Geometry check sheet. Reference: the model listing, model coordinates, mm. Coordinates: 2 decimals unless noted, no trailing zeros. Loops run counter-clockwise (first coordinate to the right, second up) from the corner with the lowest first, then second, coordinate; pieces in that order, holes last. Notation, with made-up numbers: (35.25, -6.75) - (70.25, -6.75) arc R12 ccw to (70.25, 4.25) - close; hole circle Ø11 at (36, 29). An arc over 180 degrees is marked (long way). Write item = value, one per line. Start each with the question number.
from build123d import *

# Parameters (mm, degrees)
F0_R     = 1.6
F1_DEPTH = 3.175


# Not quite as in the source:
# - a length typed as a fraction of an inch, garbled in the dataset ("3 / 203.2 mm" for 3/8 in), is restored


with BuildPart() as f1:
    # F0 (on Front) → F1 (new body)
    with BuildSketch(Plane.XZ):
        with BuildLine():
            Line((27.46, 0), (2.54, 0))
            ThreePointArc((2.54, 0), (0.7439487758, -0.7439487758), (0, -2.54))
            Line((0, -2.54), (0, -77.46))
            ThreePointArc((0, -77.46), (0.7439487758, -79.2560512242), (2.54, -80))
            Line((2.54, -80), (27.46, -80))
            ThreePointArc((27.46, -80), (29.2560512242, -79.2560512242), (30, -77.46))
            Line((30, -77.46), (30, -2.54))
            ThreePointArc((30, -2.54), (29.2560512242, -0.7439487758), (27.46, 0))
        make_face()
        with Locations((5, -75)):
            Circle(F0_R, mode=Mode.SUBTRACT)
        with Locations((5, -65)):
            Circle(F0_R, mode=Mode.SUBTRACT)
        with Locations((15, -75)):
            Circle(F0_R, mode=Mode.SUBTRACT)
        with Locations((15, -65)):
            Circle(F0_R, mode=Mode.SUBTRACT)
        with Locations((5, -55)):
            Circle(F0_R, mode=Mode.SUBTRACT)
        with Locations((5, -45)):
            Circle(F0_R, mode=Mode.SUBTRACT)
        with Locations((15, -55)):
            Circle(F0_R, mode=Mode.SUBTRACT)
        with Locations((15, -45)):
            Circle(F0_R, mode=Mode.SUBTRACT)
        with Locations((25, -75)):
            Circle(F0_R, mode=Mode.SUBTRACT)
        with Locations((25, -65)):
            Circle(F0_R, mode=Mode.SUBTRACT)
        with Locations((25, -55)):
            Circle(F0_R, mode=Mode.SUBTRACT)
        with Locations((25, -45)):
            Circle(F0_R, mode=Mode.SUBTRACT)
        with Locations((5, -35)):
            Circle(F0_R, mode=Mode.SUBTRACT)
        with Locations((5, -25)):
            Circle(F0_R, mode=Mode.SUBTRACT)
        with Locations((15, -35)):
            Circle(F0_R, mode=Mode.SUBTRACT)
        with Locations((15, -25)):
            Circle(F0_R, mode=Mode.SUBTRACT)
        with Locations((5, -15)):
            Circle(F0_R, mode=Mode.SUBTRACT)
        with Locations((5, -5)):
            Circle(F0_R, mode=Mode.SUBTRACT)
        with Locations((15, -15)):
            Circle(F0_R, mode=Mode.SUBTRACT)
        with Locations((15, -5)):
            Circle(F0_R, mode=Mode.SUBTRACT)
        with Locations((25, -35)):
            Circle(F0_R, mode=Mode.SUBTRACT)
        with Locations((25, -25)):
            Circle(F0_R, mode=Mode.SUBTRACT)
        with Locations((25, -15)):
            Circle(F0_R, mode=Mode.SUBTRACT)
        with Locations((25, -5)):
            Circle(F0_R, mode=Mode.SUBTRACT)
    extrude(amount=F1_DEPTH)


solid = f1.part
(1) Draft check along X on faces 1 (the face through (30, -2, -41)), 2 (the face through (24.65, -1.57, -36.56)), 3 (the face through (15, -3.175, -39)). Enter one of: pulls with the +X half, pulls with the -X half, needs draft (parallel to the pull), parting line crosses it, or undercut.
(2) Scan lines: line 1 (X direction, y = -1.4, z = -75); line 2 (X direction, y = -0.4, z = -66); line 3 (Z direction, x = 28.75, y = -0.75). Record each from-to range of solid material in increasing order.
(3) Sectioned sample at A-A on z = -65. Enter the section's corners in (x, y) (3 decimals).
(4) Sectioned sample at B-B on x = 15. Count the separate pieces of the cut face and the enclosed holes in it, plus the area to 3 significant figures.
(5) Depth check by flat-ended pin: pin 1 (3 mm diameter, centred on x = 25, z = -25, fed in from -Y). Enter the tip coordinate at first touch or a pass-through.
Working result:
q1.face_1 = pulls with the +X half
q1.face_2 = undercut
q1.face_3 = needs draft
q2.line_1 = 0 to 3.4, 6.6 to 13.4, 16.6 to 23.4, 26.6 to 30
q2.line_2 = 0 to 3.75, 6.25 to 13.75, 16.25 to 23.75, 26.25 to 30
q2.line_3 = -79.65 to -0.35
q3.outline = (0, -3.175) - (3.4, -3.175) - (3.4, 0) - (0, 0) - close; (6.6, -3.175) - (13.4, -3.175) - (13.4, 0) - (6.6, 0) - close; (16.6, -3.175) - (23.4, -3.175) - (23.4, 0) - (16.6, 0) - close; (26.6, -3.175) - (30, -3.175) - (30, 0) - (26.6, 0) - close
q4.separate_pieces = 9
q4.enclosed_holes = 0
q4.area = 173 mm2
q5.pin_1 = through
